Here's how the part is built. I have some questions about the finished solid (model axes, mm). A direction names the side the tool comes from. Give positions to 0.01 mm unless a question says otherwise; leave off trailing zeros. Write each loop counter-clockwise with the first axis right and the second up, starting at its lowest first coordinate (ties: lowest second). Pieces come first, ordered by that corner, then holes. Notation, with made-up numbers: (24.25, -15) -> (69.25, -15) arc R19 ccw to (69.25, 7) -> close; hole circle Ø10 at (54.5, -15). An arc over 180 degrees is marked (long way). Use one line per item in the form item = value.
```python
from build123d import *

# Parameters (mm, degrees)
PAD_DEPTH       = 19.5
POCKET_DEPTH    = 42
SKETCH003_R     = 6.4432774511
POCKET001_DEPTH = 5
SKETCH004_R     = 17.169517
POCKET002_DEPTH = 5
PAD001_DEPTH    = 40
PAD002_DEPTH    = 24
CHAMFER_SIZE    = 1


with BuildPart() as part:
    # Sketch → Pad (new body, symmetric)
    with BuildSketch(Plane.YZ):
        with BuildLine():
            Line((-24.615255, -40.645466), (-24.615255, -11.9915260199))
            Line((-24.615255, -11.9915260199), (-30.1099110656, -0.070655828))
            ThreePointArc((-29.0420891926, 3.6862219759), (-30.2710994658, 2.00535199), (-30.1099110656, -0.070655828))
            Line((-29.0420891926, 3.6862219759), (-10.21399901, 12.1607312799))
            ThreePointArc((-4.7944050935, 10.5585189909), (-7.2070537123, 12.364749952), (-10.21399901, 12.1607312799))
            Line((-4.7944050935, 10.5585189909), (9.5435566353, -19.8681705288))
            ThreePointArc((8.4289379194, -27.0849824103), (10.0898273983, -23.6470216852), (9.5435566353, -19.8681705288))
            Line((8.4289379194, -27.0849824103), (-5.794836, -34.045753))
            Line((-5.794836, -34.045753), (-5.794836, -40.645466))
            Line((-5.794836, -40.645466), (-24.615255, -40.645466))
        make_face()
        Polygon((-27.981411, 0.422502), (-27.429825, 1.92854), (-9.861721, 10.084236), (-6.402346, 8.970874), (8.119048, -22.100113), (7.085211, -25.957119), (-10.374684, -34.147896), (-12.253858, -33.776932), align=None, mode=Mode.SUBTRACT)
    extrude(amount=PAD_DEPTH, both=True)

    # Sketch002 (on Face20 of Pad) → Pocket (cut)
    with BuildSketch(Plane.YZ.offset(19.5)):
        with BuildLine():
            Line((-24.841486, -11.770947), (-14.572847112, -35.3198980182))
            ThreePointArc((-14.572847112, -35.3198980182), (-12.7694099446, -36.9511784812), (-10.3532255429, -36.6763794588))
            Line((-10.3532255429, -36.6763794588), (-4.861786, -33.667202))
            Line((-4.861786, -33.667202), (-4.861786, -40.862381))
            Line((-4.861786, -40.862381), (-24.841486, -40.862381))
            Line((-24.841486, -40.862381), (-24.841486, -11.770947))
        make_face()
    extrude(amount=-POCKET_DEPTH, mode=Mode.SUBTRACT)

    # Sketch003 (on Face13 of Pocket) → Pocket001 (cut)
    with BuildSketch(Plane(origin=(0, -6.272118922, 13.9349685583), x_dir=(0, -0.9118876327, -0.4104399412), z_dir=(0, -0.4104399412, 0.9118876327))):
        with Locations((14.81313, 0.011856)):
            Circle(SKETCH003_R)
    extrude(amount=-POCKET001_DEPTH, mode=Mode.SUBTRACT)

    # Sketch004 (on Face11 of Pocket001) → Pocket002 (cut)
    with BuildSketch(Plane(origin=(0, 0.1481790527, 0.06982638), x_dir=(0, -0.426272087, 0.9045949966), z_dir=(0, 0.9045949966, 0.426272087))):
        with Locations((-6.539624, 0)):
            Circle(SKETCH004_R)
    extrude(amount=-POCKET002_DEPTH, mode=Mode.SUBTRACT)

    # Sketch005 (on Face18 of Pocket002) → Pad001 (join)
    with BuildSketch(Plane(origin=(0, 11.2585506109, -23.9993240592), x_dir=(0, -0.9053303403, -0.4247081056), z_dir=(0, -0.4247081056, 0.9053303403))):
        Polygon((1.91594, 19.597263), (3.845239, 19.597263), (3.845239, 18.66189), (1.91594, 17.128572), align=None)
        Polygon((1.518515, -16.771593), (3.74988, -18.737337), (3.74988, -19.519863), (1.518515, -19.509285), align=None)
    extrude(amount=PAD001_DEPTH)

    # Sketch006 (on Face35 of Pad001) → Pad002 (join)
    with BuildSketch(Plane(origin=(0, -1.8135690856, -0.8475930049), x_dir=(0, 0.4234025651, -0.905941647), z_dir=(0, -0.905941647, -0.4234025651))):
        Polygon((-13.586584, 19.537718), (-11.460353, 19.537718), (-11.460353, 18.955914), (-12.613384, 17.940399), (-13.586584, 15.782431), align=None)
        Polygon((24.452187, 19.56831), (24.452187, 19.02969), (25.618814, 17.988846), (26.755948, 15.849336), (26.755948, 19.55965), align=None)
        Polygon((-13.772037, -16.08662), (-12.642, -18.040642), (-11.794474, -18.888168), (-11.818016, -19.547356), (-13.772037, -19.547356), align=None)
        Polygon((26.955989, -14.6143), (25.756637, -17.959862), (24.509941, -18.985624), (24.509941, -19.5853), (26.955989, -19.5853), align=None)
    extrude(amount=PAD002_DEPTH)

    # Chamfer
    chamfer_edges = [part.edges().sort_by_distance(p)[0] for p in [
        (0.011856, -13.904484, 10.499647),
    ]]
    chamfer(chamfer_edges, length=CHAMFER_SIZE)


solid = part.part
```
Q1. I want a section at B-B, the plane x = -15. Write out the boundary of the cut face in (y, z).
Result set:
outline = (-30.11, -0.07) -> (-24.62, -11.99) -> (-24.62, -12.29) -> (-14.57, -35.32) arc R2.95 ccw to (-10.35, -36.68) -> (-5.79, -34.18) -> (-5.79, -34.05) -> (8.43, -27.08) arc R6.53 ccw to (9.54, -19.87) -> (6.5, -13.4) -> (4.5, -14.35) -> (8.12, -22.1) -> (7.09, -25.96) -> (-10.37, -34.15) -> (-12.25, -33.78) -> (-27.98, 0.42) -> (-27.43, 1.93) -> (-9.86, 10.08) -> (-6.4, 8.97) -> (-2.58, 0.79) -> (-0.63, 1.71) -> (-4.79, 10.56) arc R4.33 ccw to (-10.21, 12.16) -> (-29.04, 3.69) arc R3 ccw to start
Q2. If we mould it in two halves opening along Z, with no side actions, what happens to faces 1 (the face through (19.597, 0, -7)), 2 (the face through (-19.12, -0.56, -7.64)), 3 (the face through (0.273, -8.106, -35.445)), 4 (the face through (5.87, -4.03, 8.94))? For each: +Z half, -Z half, draft (parallel to the pull), parting line (faces both ways), or undercut.
Result set:
face_1 = draft
face_2 = undercut
face_3 = -Z half
face_4 = +Z half
Q3. Will these pins go through, and if not, where does the flat tip stop? pin 1 Ø12 at (x, z) = (-1.5, -23) entering from -Y; pin 2 Ø6 at (y, z) = (6, -11.5) entering from +X; pin 3 Ø5 at (x, z) = (13.5, -19) entering from -Y; pin 4 Ø1.5 at (x, z) = (1, -8.5) entering from +Y.
Result set:
pin_1 = -22.56
pin_2 = 19.6
pin_3 = -22.78
pin_4 = -23.53
Q4. I want a section at C-C, the plane z = -1.5. Count the separate pieces of the cut face and the enclosed holes in it, and give its area (3 significant figures).
Result set:
separate_pieces = 3
enclosed_holes = 0
area = 113 mm2
Q5. I want a section at A-A, the plane z = -30.5. Write out the boundary of the cut face in (x, y), and give its area (3 significant figures).
Result set:
outline = (-19.59, -7.37) -> (-18.99, -7.37) -> (-17.96, -4.43) -> (-15.8, -2.6) -> (16.27, -2.6) -> (17.99, -4.75) -> (19.03, -7.51) -> (19.57, -7.51) -> (19.56, -2.07) -> (19.5, -2.07) -> (19.5, 1.45) -> (-19.5, 1.45) -> (-19.5, -1.59) -> (-19.59, -1.59) -> close; (-19.5, -16.67) -> (19.5, -16.67) -> (19.5, -13.76) -> (-19.5, -13.76) -> close
area = 288 mm2
Q6. Which directions (+Z, -Z, +X, -X, +Y, -Y) give clear straight access to the entire face, cutting with the end or side of a thin tool? Please do faces 5 (the face through (0.22, -11.301, -33.965)), 6 (the face through (-19.5, -21, -16)), 7 (the face through (0.273, -19.664, -23.644)).
Result set:
face_5 = none
face_6 = -X
face_7 = -Z, +X, -X, -Y
Q7. If I drill on line 1 along X through (y, z) = (-25.5, -10); line 2 along X through (y, z) = (2, -27); line 3 along Y through (x, z) = (-17, 0.5), over which ranges is the centre line in solid material (lowest first)? Write a range as from..to.
Result set:
line_1 = -19.5..19.5
line_2 = -19.59..-18.33, 18.27..19.57
line_3 = -30.31..-27.95, -2.44..-0.05
